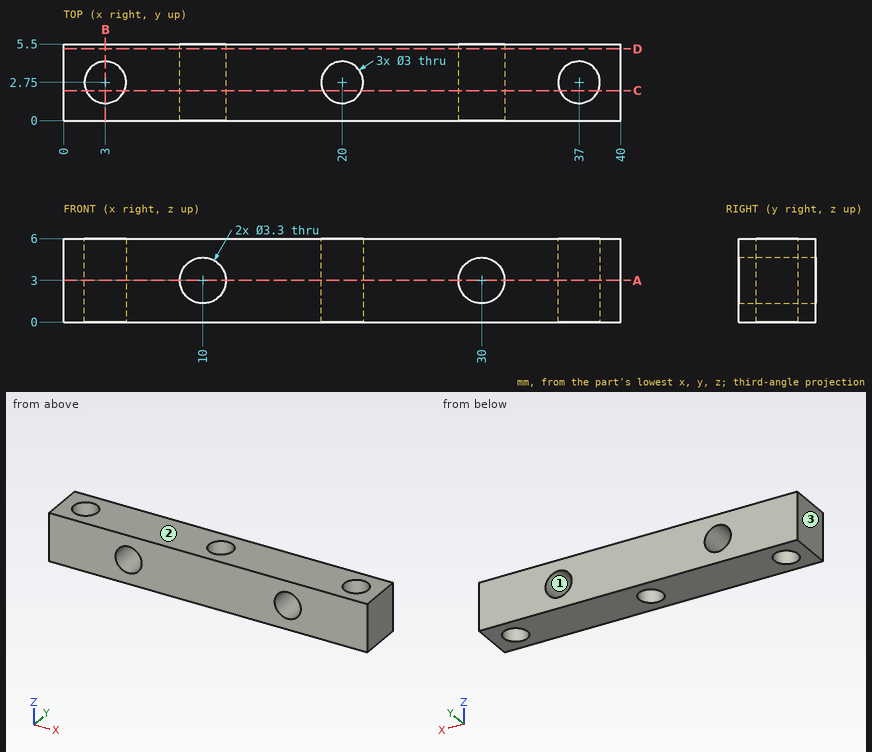
Check sheet for the drawn part. Datum: minimum x, y, z corner. Units: mm. Give positions to 0.01 mm unless a question says otherwise; leave off trailing zeros. Order: outer loops, then holes, each group sorted by start corner. A loop starts at its lowest first (then second) coordinate and runs counter-clockwise, first axis right, second up. Notation, with made-up numbers: (66.25, 59.25) - (103.25, 59.25) arc R9 cw to (103.25, 69.25) - close; hole circle Ø5 at (2.25, -32). An arc over 180 degrees is marked (long way). Write item = value, one per line. Start each with the question number.
1) Gauge pin test, flat end, axial feed: pin 1 Ø2 at (x, z) = (10, 3) entering from -Y. Record the tip position at first contact, or that the pin passes through.
2) Section check C-C (y = 2.15). Enter the section's corners in (x, z), then the cut area to 3 significant figures.
3) Scan lines: L1, parallel to Z at x = 30, y = 2.55; L2, parallel to Y at x = 20, z = 3.6; L3, parallel to X at y = 3.85, z = 3.65. Record each from-to range of solid material in increasing order.
4) Draft check along Z on the marked faces 1, 2 and 3. Enter one of: released by +Z, released by -Z, zero draft, split by the parting line, or undercut.
5) Section check D-D (y = 5.15). Enter the section's corners in (x, z), then the cut area to 3 significant figures.
6) Section check B-B (x = 3). Enter the section's corners in (y, z).
7) Section check A-A (z = 3). Enter the section's corners in (x, y).
Geometry check:
q1.pin_1 = through
q2.outline = (0, 0) - (1.63, 0) - (1.63, 6) - (0, 6) - close; (4.37, 0) - (18.63, 0) - (18.63, 6) - (4.37, 6) - close; (21.37, 0) - (35.63, 0) - (35.63, 6) - (21.37, 6) - close; (38.37, 0) - (40, 0) - (40, 6) - (38.37, 6) - close; hole circle Ø3.3 at (10, 3); hole circle Ø3.3 at (30, 3)
q2.area = 173 mm2
q3.L1 = 0 to 1.35, 4.65 to 6
q3.L2 = 0 to 1.25, 4.25 to 5.5
q3.L3 = 0 to 1.98, 4.02 to 8.48, 11.52 to 18.98, 21.02 to 28.48, 31.52 to 35.98, 38.02 to 40
q4.face_1 = undercut
q4.face_2 = released by +Z
q4.face_3 = zero draft
q5.outline = (0, 0) - (40, 0) - (40, 6) - (0, 6) - close; hole circle Ø3.3 at (10, 3); hole circle Ø3.3 at (30, 3)
q5.area = 223 mm2
q6.outline = (0, 0) - (1.25, 0) - (1.25, 6) - (0, 6) - close; (4.25, 0) - (5.5, 0) - (5.5, 6) - (4.25, 6) - close
q7.outline = (0, 0) - (8.35, 0) - (8.35, 5.5) - (0, 5.5) - close; (11.65, 0) - (28.35, 0) - (28.35, 5.5) - (11.65, 5.5) - close; (31.65, 0) - (40, 0) - (40, 5.5) - (31.65, 5.5) - close; hole circle Ø3 at (3, 2.75); hole circle Ø3 at (20, 2.75); hole circle Ø3 at (37, 2.75)
